For this review, take the finished solid that the model builds, in its own axes (mm). Face numbers are marked on the shaded views. A direction names the side the tool comes from. Round coordinates to 2 decimals unless told otherwise and drop trailing zeros. Write each loop counter-clockwise with the first axis right and the second up, starting at its lowest first coordinate (ties: lowest second). Pieces come first, ordered by that corner, then holes. Notation, with made-up numbers: M 11,-29.5 L 64,-29.5 A19 ccw 64,-5.5 Z; hole C -2,4.25 d9. An arc over 180 degrees is marked long. Answer in a Markdown table with one row per item.
Autodesk Inventor part; units mm, degrees
ref_plane "YZ Plane" through (0, 0, 0) normal (1, 0, 0) x (0, 1, 0)
ref_plane "XZ Plane" through (0, 0, 0) normal (0, 1, 0) x (-1, 0, 0)
ref_plane "XY Plane" through (0, 0, 0) normal (0, 0, 1) x (1, 0, 0)
sketch "Sketch1" plane through (0, 0, 0) normal (0, 0, 1) x (1, 0, 0)
  line L0 (12.7, -6.0198) -> (-12.7, -6.0198)
  line L1 (-12.7, -6.0198) -> (-12.7, 6.0198)
  line L2 (-12.7, 6.0198) -> (12.7, 6.0198)
  line L3 (12.7, 6.0198) -> (12.7, -6.0198)
  line L4 (12.7, -6.0198) -> (-12.7, 6.0198) construction
  line L5 (-12.7, -6.0198) -> (12.7, 6.0198) construction
  point P0 (0, 0)
  dimension "d0" = 25.4
  dimension "d1" = 12.0396
extrude "Extrusion1" add sketch "Sketch1" along normal blind 19.05
shell "Shell1" thickness 2.54 removed faces 2 at (4.2333, -2.0066, 0) at (4.2333, -2.0066, 19.05)
sketch "Sketch2" plane through (-12.7, 6.0198, 0) normal (0, 1, 0) x (1, 0, 0)
  line L0 (-2.1226, -3.175) -> (30.0619, -3.175)
  line L1 (0, 0) -> (25.4, 0)
  circle A0 centre (7.874, -3.175) radius 1.524
  circle A1 centre (17.526, -3.175) radius 1.524
  line L2 (12.7, 1.1779) -> (12.7, -16.2415)
  point P0 (12.7, 0)
  point P1 (12.7, 0)
  dimension "d23" = 3.175
  dimension "d24" = 3.048
  dimension "d25" = 9.652
extrude "Extrusion2" cut sketch "Sketch2" against normal through all
sketch "Sketch3" plane through (0, 0, 19.05) normal (0, 0, 1) x (1, 0, 0)
  line L0 (-10.16, 3.4798) -> (10.16, 3.4798)
  line L1 (10.16, 3.4798) -> (10.16, -3.4798)
  line L2 (10.16, -3.4798) -> (-10.16, -3.4798)
  line L3 (-10.16, -3.4798) -> (-10.16, 3.4798)
  line L4 (-10.16, 3.4798) -> (10.16, -3.4798) construction
  line L5 (10.16, 3.4798) -> (-10.16, -3.4798) construction
  line L6 (-12.7, 9.525) -> (12.7, 9.525)
  line L7 (15.875, 6.35) -> (15.875, -6.35)
  line L8 (12.7, -9.525) -> (-12.7, -9.525)
  line L9 (-15.875, -6.35) -> (-15.875, 6.35)
  line L10 (-15.875, 9.525) -> (15.875, -9.525) construction
  line L11 (15.875, 9.525) -> (-15.875, -9.525) construction
  arc A0 (12.7, -9.525) -> (15.875, -6.35) centre (12.7, -6.35) ccw
  arc A1 (15.875, 6.35) -> (12.7, 9.525) centre (12.7, 6.35) ccw
  arc A2 (-12.7, 9.525) -> (-15.875, 6.35) centre (-12.7, 6.35) ccw
  arc A3 (-15.875, -6.35) -> (-12.7, -9.525) centre (-12.7, -6.35) ccw
  point P0 (0, 0)
  dimension "d28" = 19.05
  dimension "d29" = 31.75
  dimension "d30" = 3.175
extrude "Extrusion3" add sketch "Sketch3" along normal blind 3.175
fillet "Fillet1" radius 3.175 4 edges at (12.7, 6.0198, 9.525) (12.7, -6.0198, 9.525) (-12.7, 6.0198, 9.525) (-12.7, -6.0198, 9.525)
properties part number "E-Stop_Fixture_Tall"
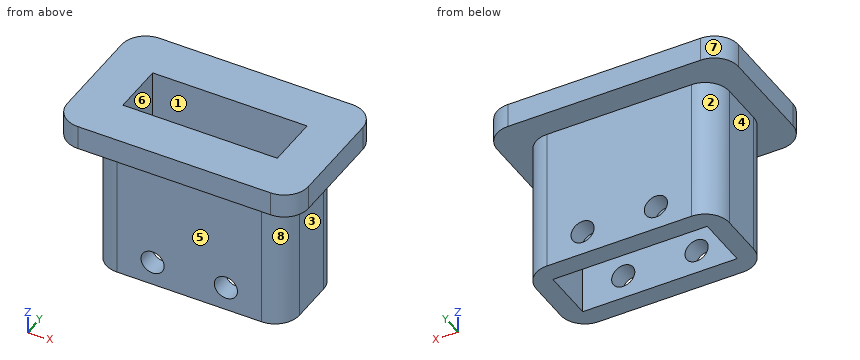
Q1. Mouldability with a two-part tool opening along Y and no side actions: class the marked faces 6, 7 and 8 as +Y half, -Y half, draft (parallel to the pull), parting line (faces both ways), or undercut.
Found:
| item | result |
|---|---|
| face 6 | undercut |
| face 7 | +Y half |
| face 8 | -Y half |
Q2. Take a section at D-D (x = -4.5). State the section outline as (y, z) points (3 decimals).
Found:
| item | result |
|---|---|
| outline | M -9.525,19.05 L -6.02,19.05 L -6.02,4.664 L -3.48,4.664 L -3.48,22.225 L -9.525,22.225 Z; M -6.02,0 L -3.48,0 L -3.48,1.686 L -6.02,1.686 Z; M 3.48,0 L 6.02,0 L 6.02,1.686 L 3.48,1.686 Z; M 3.48,4.664 L 6.02,4.664 L 6.02,19.05 L 9.525,19.05 L 9.525,22.225 L 3.48,22.225 Z |
Q3. For probe 1 along Y at (x, z) = (-3, 4.5); probe 2 along X at (y, z) = (3, 21.75) (3 decimals); probe 3 along Y at (x, z) = (-5, 20) (3 decimals), list the stretches that pass through material, from the lowest coordinate up.
Found:
| item | result |
|---|---|
| probe 1 | -6.02 to -3.48, 3.48 to 6.02 |
| probe 2 | -15.875 to -10.16, 10.16 to 15.875 |
| probe 3 | -9.525 to -3.48, 3.48 to 9.525 |
Q4. Take a section at A-A (x = 9). State the section outline as (y, z) points (3 decimals), then the cut area to 3 significant figures.
Found:
| item | result |
|---|---|
| outline | M -9.525,19.05 L -6.02,19.05 L -6.02,0 L -3.48,0 L -3.48,22.225 L -9.525,22.225 Z; M 3.48,0 L 6.02,0 L 6.02,19.05 L 9.525,19.05 L 9.525,22.225 L 3.48,22.225 Z |
| area | 135 mm² |
Q5. Machinability: for the marked faces 1, 2, 3, 4 and 5, which of the approach directions +Z, -Z, +X, -X, +Y, -Y give a long, thin tool a straight path to every point of the face, cutting with its end or side? Answer none if there is none.
Found:
| item | result |
|---|---|
| face 1 | +Z, -Z |
| face 2 | -Z, -X, +Y |
| face 3 | -Z, +X, +Y, -Y |
| face 4 | -Z, -X, +Y, -Y |
| face 5 | -Z, +X, -X, -Y |
Q6. Take a section at B-B (z = 14). State the section outline as (x, y) points (3 decimals), then the cut area to 3 significant figures.
Found:
| item | result |
|---|---|
| outline | M -12.7,-2.845 A3.175 ccw -9.525,-6.02 L 9.525,-6.02 A3.175 ccw 12.7,-2.845 L 12.7,2.845 A3.175 ccw 9.525,6.02 L -9.525,6.02 A3.175 ccw -12.7,2.845 Z; hole M -10.16,-3.48 L 10.16,-3.48 L 10.16,3.48 L -10.16,3.48 Z |
| area | 156 mm² |
Q7. Take a section at C-C (y = 5). State the section outline as (x, z) points (3 decimals), then the cut area to 3 significant figures.
Found:
| item | result |
|---|---|
| outline | M -15.875,19.05 L -11.856,19.05 L -11.856,0 L 11.856,0 L 11.856,19.05 L 15.875,19.05 L 15.875,22.225 L -15.875,22.225 Z; hole C -4.826,3.175 d3.048; hole C 4.826,3.175 d3.048 |
| area | 538 mm² |
Q8. Insertion check: P1, Ø3, axis at x = -5, z = 12.5, coming from the +Y side; P2, Ø5.5, axis at x = 0.5, z = 5, coming from the -Y side; P3, Ø5, axis at y = 1.5, z = 8, coming from the +X side. Each pin has a flat end and moves straight along its axis. Give the tip position at first contact, or say it passes through.
Found:
| item | result |
|---|---|
| P1 | y = 6.02 |
| P2 | y = -6.02 |
| P3 | x = 12.7 |
